```python
from build123d import *

# Parameters (mm, degrees)
F0_R      = 110
F1_DEPTH  = 15
F2_SIZE   = 5
F3_W      = 14.4848674536
F3_H      = 37.4039579183
F4_DEPTH  = 150
F5_R      = 5
F6_W      = 510
F6_H      = 320
F7_DEPTH  = 25
F8_SIZE   = 10
F9_R      = 2
F10_W     = 475
F10_H     = 270
F11_DEPTH = 5


with BuildPart() as f1:
    # F0 (on Top) → F1 (new body)
    with BuildSketch(Plane.XY):
        Circle(F0_R)
    extrude(amount=F1_DEPTH)

    # F2
    f2_edges = [f1.edges().sort_by_distance(p)[0] for p in [
        (-110, 0, 15),
    ]]
    chamfer(f2_edges, length=F2_SIZE)

    # F3 (on face) → F4 (join)
    with BuildSketch(Plane.XY.offset(15)):
        with Locations((0, 18.7019798905)):
            Rectangle(F3_W, F3_H)
    extrude(amount=F4_DEPTH)

    # F5
    f5_edges = [f1.edges().sort_by_distance(p)[0] for p in [
        (-7.242434, 1e-06, 90),
        (7.242434, 1e-06, 90),
        (7.242434, 37.403959, 90),
        (-7.242434, 37.403959, 90),
    ]]
    fillet(f5_edges, radius=F5_R)

    # F6 (on face) → F7 (join)
    with BuildSketch(Plane.XZ.offset(-9.313e-07)):
        with Locations((0, 240)):
            Rectangle(F6_W, F6_H)
    extrude(amount=F7_DEPTH)

    # F8
    f8_edges = [f1.edges().sort_by_distance(p)[0] for p in [
        (-255, 1e-06, 240),
        (0, 1e-06, 400),
        (255, 1e-06, 240),
    ]]
    chamfer(f8_edges, length=F8_SIZE)

    # F9
    f9_edges = [f1.edges().sort_by_distance(p)[0] for p in [
        (-255, -24.999999, 240),
        (0, -24.999999, 80),
        (255, -24.999999, 240),
        (0, -9.999999, 400),
    ]]
    fillet(f9_edges, radius=F9_R)

    # F10 (on face) → F11 (cut)
    with BuildSketch(Plane.XZ.offset(24.9999990687)):
        with Locations((0, 241)):
            Rectangle(F10_W, F10_H)
    extrude(amount=-F11_DEPTH, mode=Mode.SUBTRACT)


solid = f1.part
```
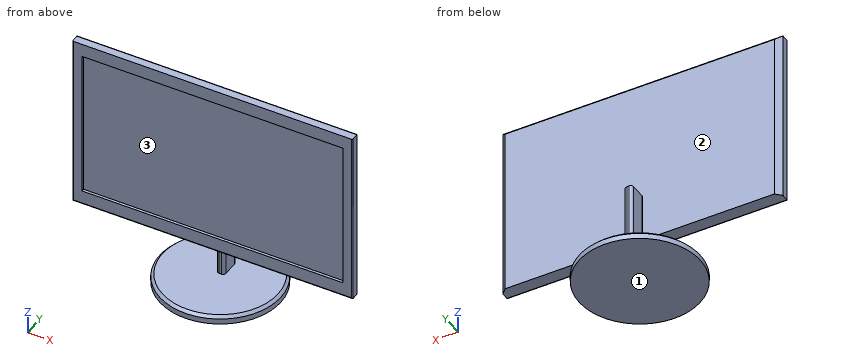
Build history of the part. All positions in model axes, mm. Face numbers are marked on the shaded views. Round coordinates to 2 decimals unless told otherwise and drop trailing zeros. Order: outer loops, then holes, each group sorted by start corner. A loop starts at its lowest first (then second) coordinate and runs counter-clockwise, first axis right, second up. Notation, with made-up numbers: (38, 7.25) -> (63, 7.25) arc R17 cw to (63, 13.25) -> close; hole circle Ø2 at (49.5, -13.75). An arc over 180 degrees is marked (long way). Answer in a Markdown table with one row per item.
1) Pin check, flat tips, straight feed: P1, Ø1.3, axis at x = 0, z = 75.5, coming from the +Y side; P2, Ø8, axis at x = -51, z = 180, coming from the +Y side; P3, Ø3.5, axis at x = 0.5, z = 51.5, coming from the -Y side. Stop position of each tip, or through.
Values:
| item | result |
|---|---|
| P1 | y = 37.4 |
| P2 | y = 0 |
| P3 | y = 0 |
2) Band-saw the part on A-A on x = 143. Give the cut face in (y, z).
Values:
| item | result |
|---|---|
| outline | (-25, 82) arc R2 ccw to (-23, 80) -> (0, 80) -> (0, 390) -> (-9.41, 399.41) arc R2 ccw to (-10.83, 400) -> (-25, 400) -> (-25, 376) -> (-20, 376) -> (-20, 106) -> (-25, 106) -> close |
3) Band-saw the part on D-D on z = 157. Give the cut face in (x, y).
Values:
| item | result |
|---|---|
| outline | (-255, -23) arc R2 ccw to (-253, -25) -> (-237.5, -25) -> (-237.5, -20) -> (237.5, -20) -> (237.5, -25) -> (253, -25) arc R2 ccw to (255, -23) -> (255, -10) -> (245, 0) -> (2.24, 0) arc R5 ccw to (7.24, 5) -> (7.24, 32.4) arc R5 ccw to (2.24, 37.4) -> (-2.24, 37.4) arc R5 ccw to (-7.24, 32.4) -> (-7.24, 5) arc R5 ccw to (-2.24, 0) -> (-245, 0) -> (-255, -10) -> close |
4) Band-saw the part on B-B on z = 60. Give the cut face in (x, y), and give its area (3 significant figures).
Values:
| item | result |
|---|---|
| outline | (-7.24, 5) arc R5 ccw to (-2.24, 0) -> (2.24, 0) arc R5 ccw to (7.24, 5) -> (7.24, 32.4) arc R5 ccw to (2.24, 37.4) -> (-2.24, 37.4) arc R5 ccw to (-7.24, 32.4) -> close |
| area | 520 mm2 |
5) Wall check: L1, parallel to Z at x = -77, y = -18.5; L2, parallel to Y at x = -136.5, z = 151.5; L3, parallel to Y at x = 162.5, z = 377. Give the ranges that are in metal, low to high.
Values:
| item | result |
|---|---|
| L1 | 0 to 15, 80 to 400 |
| L2 | -20 to 0 |
| L3 | -25 to 0 |
6) Mould opens along Z. For the marked faces 1, 2 and 3 say: released by +Z, released by -Z, zero draft, split by the parting line, or undercut.
Values:
| item | result |
|---|---|
| face 1 | released by -Z |
| face 2 | zero draft |
| face 3 | undercut |
7) Band-saw the part on C-C on z = 200. Give the cut face in (x, y), and give its area (3 significant figures).
Values:
| item | result |
|---|---|
| outline | (-255, -23) arc R2 ccw to (-253, -25) -> (-237.5, -25) -> (-237.5, -20) -> (237.5, -20) -> (237.5, -25) -> (253, -25) arc R2 ccw to (255, -23) -> (255, -10) -> (245, 0) -> (-245, 0) -> (-255, -10) -> close |
| area | 10,300 mm2 |
